Model file for the job. Use its own axes, mm. A direction names the side the tool comes from. Coordinates: 2 decimals unless noted, no trailing zeros. Write each loop counter-clockwise with the first axis right and the second up, starting at its lowest first coordinate (ties: lowest second). Pieces come first, ordered by that corner, then holes.
Q1. Pull direction Y, two halves, no side cores. Call faces 1 (the flat face through (-30, 2.4, 2.4)), 2 (the cylindrical face through (-28, -6, 0)), 3 (the flat face through (-5, 0, 0)): released by +Y, released by -Y, zero draft, split by the parting line, or undercut.
Q2. Drill centre lines: probe 1 along Z at (x, y) = (-14.75, 0); probe 2 along Z at (x, y) = (-25.75, -1). Where is each one in solid material? Low to high.
Q3. Pin check, flat tips, straight feed: P1, Ø4, axis at x = -21, z = 2.5, coming from the +Y side; P2, Ø3, axis at x = -13, y = 3, coming from the +Z side; P3, Ø1, axis at x = -22.5, y = -2, coming from the -Z side. Stop position of each tip, or through.
Q4. Which spindle directions (+Z, -Z, +X, -X, +Y, -Y) get a long thin tool onto all of the face, cutting with end or side? Do faces 4 (the cylindrical face through (-17.08, -0.54, 2.44)), 5 (the flat face through (0, 0, 0)), 6 (the flat face through (-25, 5, 0)). Say none if no direction does.
Q5. Band-saw the part on D-D, the plane x = -3.5. Write the cut outline in (y, z), plus the area to 3 significant figures.
Q6. Band-saw the part on C-C, the plane x = -14.75. Write the cut outline in (y, z).
Q7. Band-saw the part on A-A, the plane y = 0. Write the cut outline in (x, z), plus the area to 3 significant figures.
from build123d import *

# Parameters (mm, degrees)
CHAFL_N1_SIZE = 0.5
REDONDEO1_R   = 0.5


with BuildPart() as part:
    # Croquis1 → Revolución1 (revolve)
    with BuildSketch(Plane.XY):
        Polygon((0, 0), (0, 4), (-25, 4), (-25, 6), (-30, 6), (-30, 2.5), (-5, 2.5), (-5, 0), align=None)
    revolve(axis=Axis((0, 0, 0), (-1, 0, 0)))

    # Chaflán1
    chafl_n1_edges = [part.edges().sort_by_distance(p)[0] for p in [
        (-30, -2.5, 0),
        (0, -4, 0),
    ]]
    chamfer(chafl_n1_edges, length=CHAFL_N1_SIZE)

    # Redondeo1
    redondeo1_edges = [part.edges().sort_by_distance(p)[0] for p in [
        (-30, -6, 0),
        (-25, -6, 0),
        (-25, -4, 0),
    ]]
    fillet(redondeo1_edges, radius=REDONDEO1_R)


solid = part.part
Answer sheet:
1. face 1: zero draft
1. face 2: split by the parting line
1. face 3: undercut
2. probe 1: z = -4 to -2.5, 2.5 to 4
2. probe 2: z = -5.92 to -2.29, 2.29 to 5.92
3. P1: stops at y = 3.97
3. P2: stops at z = 3.71
3. P3: stops at z = -3.71
4. face 4: -X
4. face 5: +Z, -Z, +X, +Y, -Y
4. face 6: +X
5. outline: circle Ø8 at (0, 0)
5. area: 50.3 mm2
6. outline: circle Ø8 at (0, 0); hole circle Ø5 at (0, 0)
7. outline: (-30, -5.5) arc R0.5 ccw to (-29.5, -6) - (-25.5, -6) arc R0.5 ccw to (-25, -5.5) - (-25, -4.5) arc R0.5 cw to (-24.5, -4) - (-0.5, -4) - (0, -3.5) - (0, 3.5) - (-0.5, 4) - (-24.5, 4) arc R0.5 cw to (-25, 4.5) - (-25, 5.5) arc R0.5 ccw to (-25.5, 6) - (-29.5, 6) arc R0.5 ccw to (-30, 5.5) - (-30, 3) - (-29.5, 2.5) - (-5, 2.5) - (-5, -2.5) - (-29.5, -2.5) - (-30, -3) - close
7. area: 134 mm2
